```python
from build123d import *

# Parameters (mm, degrees)
EXTRUDE_THIN1_DEPTH = 100
SKETCH2_R           = 2.5
CUT_EXTRUDE1_DEPTH  = 10
SKETCH3_R           = 2.5
CUT_EXTRUDE2_DEPTH  = 10


with BuildPart() as part:
    # Sketch1 → Extrude-Thin1 (new body)
    with BuildSketch(Plane(origin=(0, 0, 0), x_dir=(1, 0, 0), z_dir=(0, 1, 0))):
        Polygon((-16.299038106, 25.230762114), (-0.866025404, -1.5), (30, -1.5), (30, 1.5), (0.866025404, 1.5), (-13.700961894, 26.730762114), align=None)
    extrude(amount=EXTRUDE_THIN1_DEPTH)

    # Sketch2 → Cut-Extrude1 (cut)
    with BuildSketch(Plane(origin=(1.299038106, 0, -0.75), x_dir=(-0.5, 0, -0.866025404), z_dir=(0.866025404, 0, -0.5))):
        with Locations((11.866025404, 90)):
            Circle(SKETCH2_R)
        with Locations((11.866025404, 50)):
            Circle(SKETCH2_R)
        with Locations((11.866025404, 10)):
            Circle(SKETCH2_R)
    extrude(amount=-CUT_EXTRUDE1_DEPTH, mode=Mode.SUBTRACT)

    # Sketch3 → Cut-Extrude2 (cut)
    with BuildSketch(Plane(origin=(0, 0, -1.5), x_dir=(-1, 0, 0), z_dir=(0, 0, -1))):
        with Locations((-15.433012702, 50)):
            Circle(SKETCH3_R)
        with Locations((-15.433012702, 10)):
            Circle(SKETCH3_R)
        with Locations((-15.433012702, 90)):
            Circle(SKETCH3_R)
    extrude(amount=-CUT_EXTRUDE2_DEPTH, mode=Mode.SUBTRACT)


solid = part.part
```
Check sheet for the modelled part. Datum: model origin and axes. Units: mm. A direction names the side the tool comes from. Give positions to 0.01 mm unless a question says otherwise; leave off trailing zeros. Order: outer loops, then holes, each group sorted by start corner. A loop starts at its lowest first (then second) coordinate and runs counter-clockwise, first axis right, second up. Notation, with made-up numbers: (27.5, -20.75) -> (66.5, -20.75) arc R11 cw to (66.5, -14.75) -> close; hole circle Ø1 at (7, 40). An arc over 180 degrees is marked (long way). Return JSON: item names as keys, results as strings.
1. Set-up check for faces 1 (the flat face through (-14.98, 49.3, -25.99)), 2 (the flat face through (19, 49, -1.5)): record each of +Z, -Z, +X, -X, +Y, -Y from which the full face is reachable in a straight line by a thin tool's end or side.
From the geometry:
{"face 1": "-Z, -X, +Y, -Y", "face 2": "-Z, +X, +Y, -Y"}
2. Mould release check, pull along Y, two halves, no side actions. Record for faces 3 (the cylindrical face through (17.42, 8.48, -0.02)), 4 (the flat face through (11, 49, 1.5)), 5 (the flat face through (3, 0, -1)), 6 (the cylindrical face through (-5.75, 92.48, -10)): +Y half, -Y half, draft (parallel to the pull), parting line (faces both ways), or undercut.
From the geometry:
{"face 3": "undercut", "face 4": "draft", "face 5": "-Y half", "face 6": "undercut"}
3. Cross-section at A-A, the plane y = 10. Record the cut outline in (x, z).
From the geometry:
{"outline": "(-16.3, -25.23) -> (-13.7, -26.73) -> (-5.88, -13.19) -> (-8.48, -11.69) -> close; (-5.98, -7.36) -> (-3.38, -8.86) -> (0.87, -1.5) -> (12.93, -1.5) -> (12.93, 1.5) -> (-0.87, 1.5) -> close; (17.93, -1.5) -> (30, -1.5) -> (30, 1.5) -> (17.93, 1.5) -> close"}
4. Cross-section at B-B, the plane x = 25.5. Record the cut outline in (y, z), plus the area to 3 significant figures.
From the geometry:
{"outline": "(0, -1.5) -> (100, -1.5) -> (100, 1.5) -> (0, 1.5) -> close", "area": "300 mm^2"}
5. Cross-section at C-C, the plane y = 41.5. Record the cut outline in (x, z), plus the area to 3 significant figures.
From the geometry:
{"outline": "(-16.3, -25.23) -> (-13.7, -26.73) -> (0.87, -1.5) -> (30, -1.5) -> (30, 1.5) -> (-0.87, 1.5) -> close", "area": "180 mm^2"}
6. Material ranges on probe 1 along Z at (x, y) = (8, 81); probe 2 along Z at (x, y) = (-2.5, 35); probe 3 along X at (y, z) = (35.5, -16), recorded low to high. Write a range as [from, to].
From the geometry:
{"probe 1": "[-1.5, 1.5]", "probe 2": "[-7.33, -1.33]", "probe 3": "[-10.97, -7.51]"}
7. Go/stop test with flat-tipped pins: P1, Ø8, axis at x = -7.5, y = 73, coming from the +Z side; P2, Ø6, axis at y = 85.5, z = -17, coming from the -X side; P3, Ø2, axis at y = 75, z = -13, coming from the +X side; P4, Ø4, axis at x = 15.43, y = 90, coming from the -Z side. Record where each tip stops, or that it passes through.
From the geometry:
{"P1": "z = -3.06", "P2": "x = -13.28", "P3": "x = -5.2", "P4": "through"}
8. Cross-section at D-D, the plane z = -23.5. Record the cut outline in (x, y).
From the geometry:
{"outline": "(-15.3, 0) -> (-11.84, 0) -> (-11.84, 100) -> (-15.3, 100) -> close"}
